from build123d import *

# Parameters (mm, degrees)
F0_W     = 15
F0_H     = 15
F1_DEPTH = 2
F3_DEPTH = 3.5


with BuildPart() as f1:
    # F0 (on Top) → F1 (new body)
    with BuildSketch(Plane.XY):
        Rectangle(F0_W, F0_H)
    extrude(amount=F1_DEPTH)

    # F2 (on face) → F3 (join)
    with BuildSketch(Plane.XY.offset(2)):
        Polygon((-3.4, -2), (-0.75, -2), (-0.75, -0.75), (-2.125, -0.75), (-2.125, 0.75), (-0.75, 0.75), (-0.75, 2), (-3.4, 2), align=None)
        Polygon((0.75, -2), (3.4, -2), (3.4, 2), (0.75, 2), (0.75, 0.75), (2.125, 0.75), (2.125, -0.75), (0.75, -0.75), align=None)
    extrude(amount=F3_DEPTH)


solid = f1.part
CAD build for the part. Positions are in the model's coordinates, mm. A direction names the side the tool comes from. Coordinates: 2 decimals unless noted, no trailing zeros. Write each loop counter-clockwise with the first axis right and the second up, starting at its lowest first coordinate (ties: lowest second). Pieces come first, ordered by that corner, then holes. Notation, with made-up numbers: M 48.25,34 L 75.25,34 A33 cw 75.25,65 Z; hole C 43,-13.5 d5. An arc over 180 degrees is marked long. Answer as a JSON object with one key per item and string values. Group by question number.
1) Mould opens along X. For faces 1 (the face through (-2, -2, 4)), 2 (the face through (-7.5, 0, 1)), 3 (the face through (-1, 0.75, 4)) say: +X half, -X half, draft (parallel to the pull), parting line (faces both ways), or undercut.
2) Saw through at D-D (x = 6.5). Write the cut outline in (y, z), plus the area to 3 significant figures.
3) Pin check, flat tips, straight feed: pin 1 Ø1 at (y, z) = (-1.5, 3.5) entering from +X; pin 2 Ø1.5 at (x, z) = (1, 3) entering from +Y; pin 3 Ø2 at (y, z) = (4.5, 4) entering from -X; pin 4 Ø3 at (x, y) = (0.5, -4.5) entering from +Z. Stop position of each tip, or through.
4) Saw through at C-C (y = 1.75). Write the cut outline in (x, z).
5) Tool access for faces 4 (the face through (0.75, 1, 4)), 5 (the face through (-3.4, 0, 4)), 6 (the face through (-2.125, 0, 4)): list every direction of +Z, -Z, +X, -X, +Y, -Y with a clear straight run to the whole face (end or side of a thin tool).
6) Saw through at B-B (x = -1.75). Write the cut outline in (y, z), plus the area to 4 significant figures.
7) Wall check: line 1 (Y direction, x = -2, z = 2.6); line 2 (X direction, y = -0.25, z = 3.15) (3 decimals); line 3 (X direction, y = 1, z = 4.05). Give the ranges that are in metal, low to high. Write a range as from..to.
8) Saw through at A-A (z = 2.2). Write the cut outline in (x, y) (3 decimals).
Values follow:
{
 "1": {"face 1": "draft", "face 2": "-X half", "face 3": "undercut"},
 "2": {"outline": "M -7.5,0 L 7.5,0 L 7.5,2 L -7.5,2 Z", "area": "30.0 mm2"},
 "3": {"pin 1": "stops at x = 3.4", "pin 2": "stops at y = 2", "pin 3": "passes through", "pin 4": "stops at z = 2"},
 "4": {"outline": "M -7.5,0 L 7.5,0 L 7.5,2 L 3.4,2 L 3.4,5.5 L 0.75,5.5 L 0.75,2 L -0.75,2 L -0.75,5.5 L -3.4,5.5 L -3.4,2 L -7.5,2 Z"},
 "5": {"face 4": "+Z, +Y, -Y", "face 5": "+Z, -X, +Y, -Y", "face 6": "+Z"},
 "6": {"outline": "M -7.5,0 L 7.5,0 L 7.5,2 L 2,2 L 2,5.5 L 0.75,5.5 L 0.75,2 L -0.75,2 L -0.75,5.5 L -2,5.5 L -2,2 L -7.5,2 Z", "area": "38.75 mm2"},
 "7": {"line 1": "y = -2..-0.75, 0.75..2", "line 2": "x = -3.4..-2.125, 2.125..3.4", "line 3": "x = -3.4..-0.75, 0.75..3.4"},
 "8": {"outline": "M -3.4,-2 L -0.75,-2 L -0.75,-0.75 L -2.125,-0.75 L -2.125,0.75 L -0.75,0.75 L -0.75,2 L -3.4,2 Z; M 0.75,-2 L 3.4,-2 L 3.4,2 L 0.75,2 L 0.75,0.75 L 2.125,0.75 L 2.125,-0.75 L 0.75,-0.75 Z"}
}
